Can you work these out from the drawing? Everything is in mm from the part's minimum corner. Give positions to 0.01 mm unless a question says otherwise; leave off trailing zeros. Write each loop counter-clockwise with the first axis right and the second up, starting at its lowest first coordinate (ties: lowest second). Pieces come first, ordered by that corner, then holes. Notation, with made-up numbers: (-19, 78) - (37, 78) arc R19 cw to (37, 84) - close; hole circle Ø5 at (63, 2). An arc over 180 degrees is marked (long way). Use a Markdown table: item, result. Add a question column.
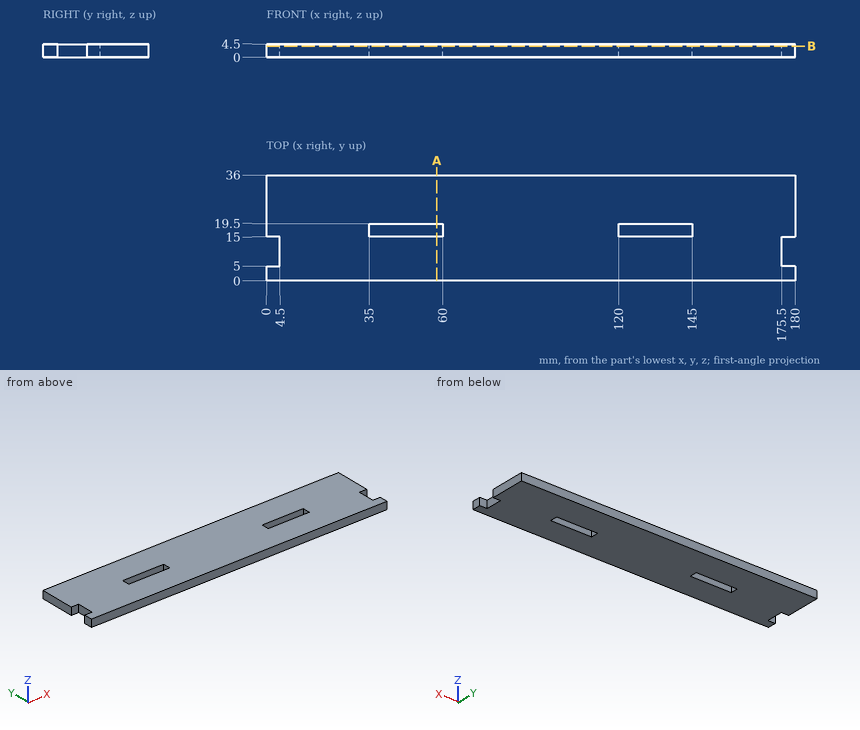
Q1. I'm going to push flat-ended pins straight in: P1, Ø1.3, axis at y = 10.5, z = 3, coming from the +X side; P2, Ø1.3, axis at x = 133.5, z = 3.5, coming from the -Y side. Where does each tip first touch, or does it pass through?
Q2. Suppose I cut it at B-B (z = 3.8). Please give me the cut outline in (x, y), and give its area (4 significant figures).
Q3. If I drill on probe 1 along X at (y, z) = (19, 2.65); probe 2 along Y at (x, z) = (125.5, 2.6); probe 3 along X at (y, z) = (11, 3.55), over which ranges is the centre line in solid material (lowest first)? Write a range as [from, to].
Q4. Suppose I cut it at A-A (x = 58). Please give me the cut outline in (y, z), and give its area (3 significant figures).
Derived:
| question | item | result |
|---|---|---|
| 1 | P1 | x = 175.5 |
| 1 | P2 | y = 0 |
| 2 | outline | (0, 0) - (180, 0) - (180, 5) - (175.5, 5) - (175.5, 15) - (180, 15) - (180, 36) - (0, 36) - (0, 15) - (4.5, 15) - (4.5, 5) - (0, 5) - close; hole (35, 15) - (60, 15) - (60, 19.5) - (35, 19.5) - close; hole (120, 15) - (145, 15) - (145, 19.5) - (120, 19.5) - close |
| 2 | area | 6,165 mm² |
| 3 | probe 1 | [0, 35], [60, 120], [145, 180] |
| 3 | probe 2 | [0, 15], [19.5, 36] |
| 3 | probe 3 | [4.5, 175.5] |
| 4 | outline | (0, 0) - (15, 0) - (15, 4.5) - (0, 4.5) - close; (19.5, 0) - (36, 0) - (36, 4.5) - (19.5, 4.5) - close |
| 4 | area | 142 mm² |
